from build123d import *

# Parameters (mm, degrees)
F0_W     = 100
F0_H     = 100
F1_DEPTH = 100
F2_W     = 100
F2_H     = 100
F3_DEPTH = 40
F4_W     = 60
F4_H     = 40
F5_DEPTH = 176
F6_W     = 60
F6_H     = 40
F7_DEPTH = 223


with BuildPart() as f1:
    # F0 (on Top) → F1 (new body)
    with BuildSketch(Plane.XY):
        Rectangle(F0_W, F0_H)
    extrude(amount=F1_DEPTH)

    # F2 (on face) → F3 (cut)
    with BuildSketch(Plane.XY.offset(100)):
        Rectangle(F2_W, F2_H)
    extrude(amount=-F3_DEPTH, mode=Mode.SUBTRACT)

    # F4 (on face) → F5 (cut)
    with BuildSketch(Plane.XZ.offset(50)):
        with Locations((-0.226441, 20)):
            Rectangle(F4_W, F4_H)
    extrude(amount=-F5_DEPTH, mode=Mode.SUBTRACT)

    # F6 (on face) → F7 (cut)
    with BuildSketch(Plane(origin=(-50, 0, 0), x_dir=(0, -1, 0), z_dir=(-1, 0, 0))):
        with Locations((5.599647, 20)):
            Rectangle(F6_W, F6_H)
    extrude(amount=-F7_DEPTH, mode=Mode.SUBTRACT)


solid = f1.part
The model under review builds one solid part; all positions refer to its coordinate system, in mm. A direction names the side the tool comes from. Coordinates: 2 decimals unless noted, no trailing zeros. Loops run counter-clockwise (first coordinate to the right, second up) from the corner with the lowest first, then second, coordinate; pieces in that order, holes last.
(1) Consider section D-D, the plane y = 5. Give the boundary of the cut face in (x, z), plus the area to 3 significant figures.
Determined:
outline: (-50, 40) - (50, 40) - (50, 60) - (-50, 60) - close
area: 2,000 mm2
(2) Consider section B-B, the plane x = -33. Give the boundary of the cut face in (y, z).
Determined:
outline: (-50, 0) - (-35.6, 0) - (-35.6, 40) - (24.4, 40) - (24.4, 0) - (50, 0) - (50, 60) - (-50, 60) - close
(3) Wall thickness on L1, parallel to X at y = -43.5, z = 9.5; L2, parallel to Z at x = -29, y = -8: over which ranges is each line inside the solid? List them lowest first.
Determined:
L1: x = -50 to -30.23, 29.77 to 50
L2: z = 40 to 60
(4) Draft analysis for pull direction X (two halves, no side actions). For faces 4 (the flat face through (-50, -1, 43)), 5 (the flat face through (50, -1, 43)), 6 (the flat face through (29.774, 37, 20)), state which applies: +X half, -X half, draft (parallel to the pull), parting line (faces both ways), or undercut.
Determined:
face 4: -X half
face 5: +X half
face 6: undercut
(5) Consider section A-A, the plane z = 29. Give the boundary of the cut face in (x, y), plus the area to 3 significant figures.
Determined:
outline: (-50, -50) - (-30.23, -50) - (-30.23, -35.6) - (-50, -35.6) - close; (-50, 24.4) - (-30.23, 24.4) - (-30.23, 50) - (-50, 50) - close; (29.77, -50) - (50, -50) - (50, -35.6) - (29.77, -35.6) - close; (29.77, 24.4) - (50, 24.4) - (50, 50) - (29.77, 50) - close
area: 1,600 mm2
(6) Insertion check: P1, Ø10, axis at x = -15.5, y = -32.5, coming from the -Z side. The pin has a flat end and moves straight along its axis. Give the tip position at first contact, or say it passes through.
Determined:
P1: stops at z = 40
(7) Tool access review of faces 1 (the flat face through (40, 24.4, 20)), 2 (the flat face through (-40, -43, 0)), 3 (the flat face through (-30.226, -43, 20)): name each direction out of +Z, -Z, +X, -X, +Y, -Y from which nothing blocks a thin tool from reaching the whole face with its end or side.
Determined:
face 1: -Z, +X, -X
face 2: -Z, +X, -X, +Y, -Y
face 3: -Z, +Y, -Y
(8) Consider section C-C, the plane y = 36. Give the boundary of the cut face in (x, z), plus the area to 3 significant figures.
Determined:
outline: (-50, 0) - (-30.23, 0) - (-30.23, 40) - (29.77, 40) - (29.77, 0) - (50, 0) - (50, 60) - (-50, 60) - close
area: 3,600 mm2
